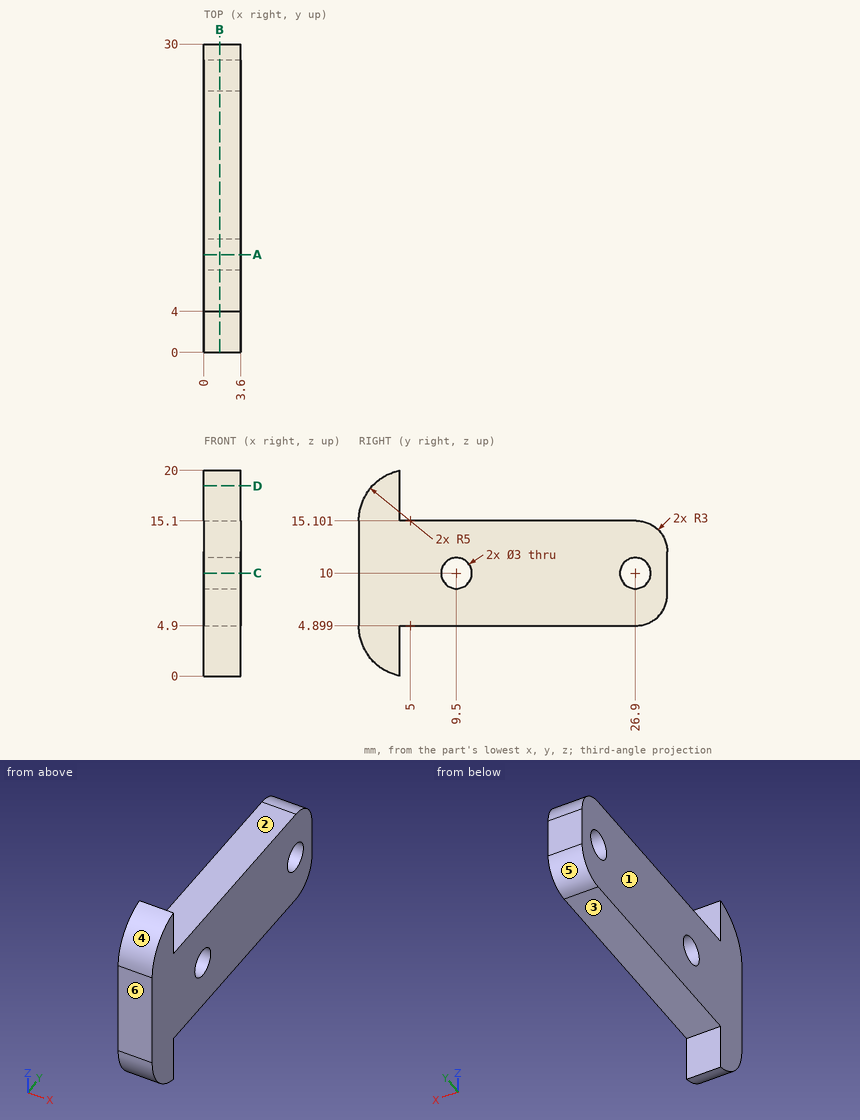
Check sheet for the drawn part. Datum: minimum x, y, z corner. Units: mm. A direction names the side the tool comes from. Round coordinates to 2 decimals unless told otherwise and drop trailing zeros. Order: outer loops, then holes, each group sorted by start corner. A loop starts at its lowest first (then second) coordinate and runs counter-clockwise, first axis right, second up. Notation, with made-up numbers: M 78,-33 L 105,-33 A14 cw 105,-13 Z; hole C 86,-39.5 d1. An arc over 180 degrees is marked long. Write each question's results on one line, items separated by ' | '. Start each with the question number.
1. Draft check along Z on the marked faces 4, 5 and 6. Enter one of: pulls with the +Z half, pulls with the -Z half, needs draft (parallel to the pull), parting line crosses it, or undercut.
2. Cross-section at B-B on x = 1.55. Record the boundary of the cut face in (y, z).
3. Cross-section at C-C on z = 10. Record the boundary of the cut face in (x, y), plus the area to 3 significant figures.
4. Set-up check for the marked faces 1, 2 and 3: record each of +Z, -Z, +X, -X, +Y, -Y from which the full face is reachable in a straight line by a thin tool's end or side.
5. Cross-section at A-A on y = 9.5. Record the boundary of the cut face in (x, z), plus the area to 3 significant figures.
6. Go/stop test with flat-tipped pins: P1, Ø1, axis at x = 2.5, y = 7, coming from the -Z side; P2, Ø1, axis at x = 2.5, z = 14.5, coming from the +Y side; P3, Ø1.1, axis at x = 2.5, z = 2, coming from the +Y side. Record where each tip stops, or that it passes through.
7. Material ranges on L1, parallel to Y at x = 0.8, z = 10; L2, parallel to Y at x = 1.9, z = 8.75; L3, parallel to Z at x = 1.05, y = 16, recorded low to high. Write a range as from..to.
8. Cross-section at D-D on z = 18.5. Record the boundary of the cut face in (x, y).
Resolved:
1) face 4: pulls with the +Z half | face 5: pulls with the -Z half | face 6: needs draft
2) outline: M 0,4.9 A5 ccw 4,0 L 4,4.9 L 27,4.9 A3 ccw 30,7.9 L 30,12.1 A3 ccw 27,15.1 L 4,15.1 L 4,20 A5 ccw 0,15.1 Z; hole C 9.5,10 d3; hole C 26.9,10 d3
3) outline: M 0,0 L 3.6,0 L 3.6,8 L 0,8 Z; M 0,11 L 3.6,11 L 3.6,25.4 L 0,25.4 Z; M 0,28.4 L 3.6,28.4 L 3.6,30 L 0,30 Z | area: 86.4 mm2
4) face 1: +Z, -Z, -X, +Y, -Y | face 2: +Z, +X, -X, +Y | face 3: -Z, +X, -X, +Y
5) outline: M 0,4.9 L 3.6,4.9 L 3.6,8.5 L 0,8.5 Z; M 0,11.5 L 3.6,11.5 L 3.6,15.1 L 0,15.1 Z | area: 25.9 mm2
6) P1: z = 4.9 | P2: y = 29.32 | P3: y = 4
7) L1: 0..8, 11..25.4, 28.4..30 | L2: 0..8.67, 10.33..26.07, 27.73..30 | L3: 4.9..15.1
8) outline: M 0,1.33 L 3.6,1.33 L 3.6,4 L 0,4 Z
